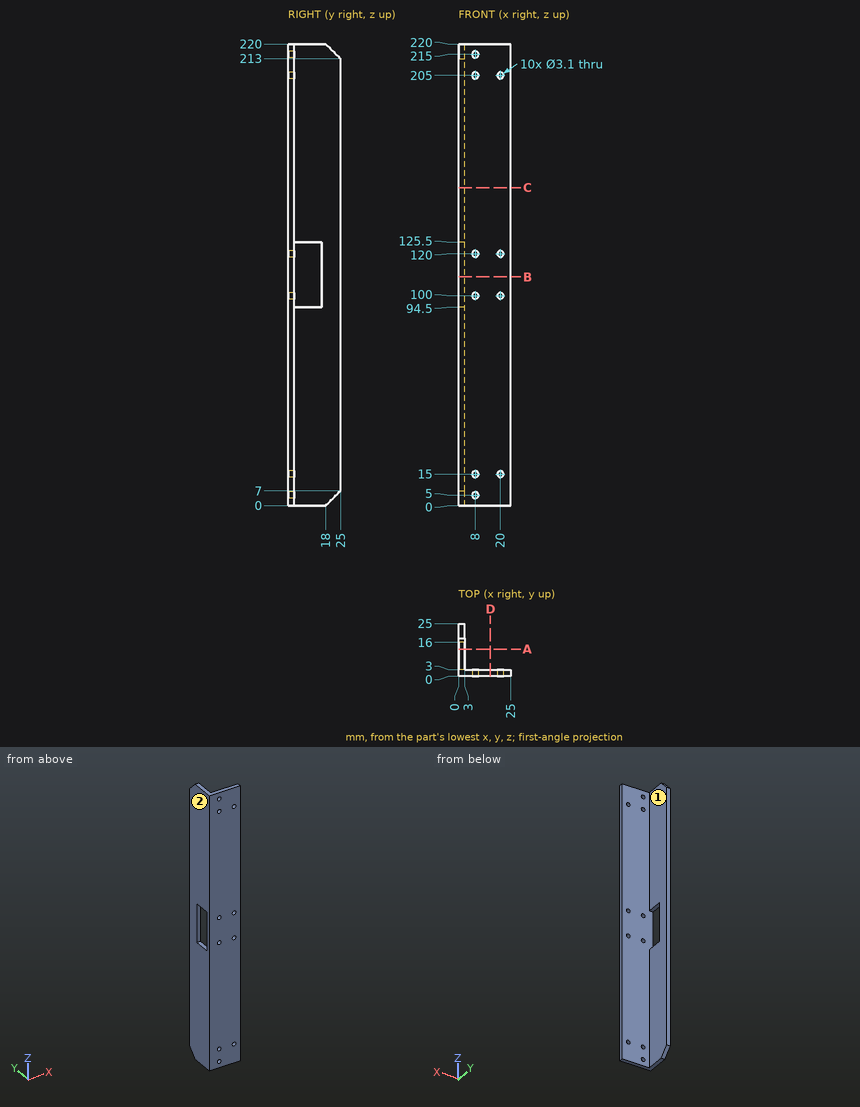
Study the drawing (mm; zero at the part's minimum x, y, z) and answer. A direction names the side the tool comes from. Round coordinates to 2 decimals unless told otherwise and drop trailing zeros. Order: outer loops, then holes, each group sorted by start corner. A loop starts at its lowest first (then second) coordinate and runs counter-clockwise, first axis right, second up. Notation, with made-up numbers: M 21,-38.75 L 57,-38.75 A21 cw 57,-19.75 Z; hole C 77.5,4 d5. An arc over 180 degrees is marked long. One line per item, written item: value.
Q1. Find section D-D on x = 15.25. Write down the section's boundary in (y, z).
Derived:
outline: M 0,0 L 3,0 L 3,220 L 0,220 Z
Q2. Find section A-A on y = 12.75. Write down the section's boundary in (x, z).
Derived:
outline: M 0,0 L 3,0 L 3,94.5 L 0,94.5 Z; M 0,125.5 L 3,125.5 L 3,220 L 0,220 Z
Q3. Straight lines are drawn through the part: line 1 (X direction, y = 1.7, z = 120); line 2 (Y direction, x = 2, z = 124.5); line 3 (Y direction, x = 23.25, z = 120.5). For each, find the intervals that lie inside material, in ascending order.
Derived:
line 1: 0 to 6.45, 9.55 to 18.45, 21.55 to 25
line 2: 0 to 3, 16 to 25
line 3: 0 to 3
Q4. Find section B-B on z = 109. Write down the section's boundary in (x, y).
Derived:
outline: M 0,0 L 25,0 L 25,3 L 0,3 Z; M 0,16 L 3,16 L 3,25 L 0,25 Z
Q5. Flat-ended cylindrical pins translate along their axes: pin 1 (5 mm diameter, centred on x = 8, z = 120, fed in from +Y); pin 2 (6 mm diameter, centred on y = 16, z = 181.5, fed in from +X); pin 3 (10 mm diameter, centred on y = 10, z = 66, fed in from -X). Find the tip coordinate at first contact, or state that the pin passes through.
Derived:
pin 1: y = 3
pin 2: x = 3
pin 3: x = 0
Q6. For the marked faces 1 and 2, determine the directions among +Z, -Z, +X, -X, +Y, -Y from which every point of the face is accessible in a straight line to the end or side of a thin tool.
Derived:
face 1: +Z, -Z, +X, +Y
face 2: +Z, -Z, -X, +Y, -Y
Q7. Find section C-C on z = 151.5. Write down the section's boundary in (x, y).
Derived:
outline: M 0,0 L 25,0 L 25,3 L 3,3 L 3,25 L 0,25 Z
